Part model, mm, in its own coordinate system. Give positions to 0.01 mm unless a question says otherwise; leave off trailing zeros. Order: outer loops, then holes, each group sorted by start corner. A loop starts at its lowest first (then second) coordinate and runs counter-clockwise, first axis right, second up.
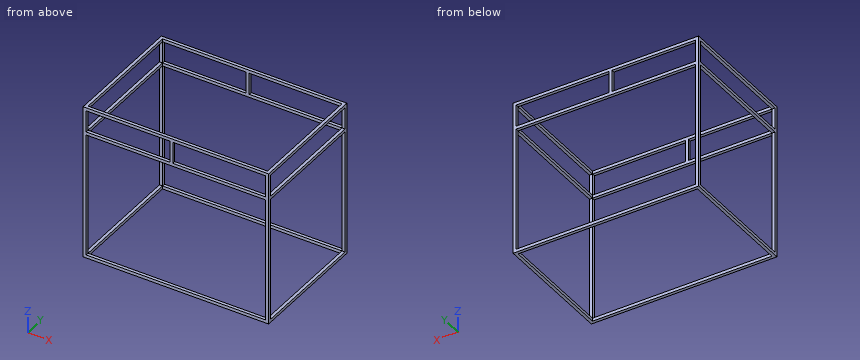
from build123d import *

# Parameters (mm, degrees)
SKETCH1_W               = 914.4
SKETCH1_H               = 609.6
SKETCH1_W_2             = 884.4
SKETCH1_H_2             = 579.6
BOSS_EXTRUDE2_DEPTH     = 762
SKETCH4_W               = 884.4
SKETCH4_H               = 609.6
SKETCH4_W_2             = 412.2
SKETCH4_H_2             = 107.4
SKETCH4_W_3             = 457.2
CUT_EXTRUDE3_DEPTH      = 762
CUT_EXTRUDE4_DEPTH      = 1374.291942344
CUT_EXTRUDE4_DEPTH_BACK = 1374.291942344
SKETCH5_W               = 107.4
SKETCH5_H               = 579.6
SKETCH5_W_2             = 609.6


with BuildPart() as part:
    # Sketch1 → Boss-Extrude2 (new body)
    with BuildSketch(Plane.XY):
        with Locations((479.545925455, 380.152114317)):
            Rectangle(SKETCH1_W, SKETCH1_H)
        with Locations((479.545925455, 380.152114317)):
            Rectangle(SKETCH1_W_2, SKETCH1_H_2, mode=Mode.SUBTRACT)
    extrude(amount=BOSS_EXTRUDE2_DEPTH)

    # Sketch4 → Cut-Extrude3 (cut)
    with BuildSketch(Plane(origin=(0, 75.352114317, 0), x_dir=(-1, 0, 0), z_dir=(0, -1, 0))):
        with Locations((-479.545925455, -319.8)):
            Rectangle(SKETCH4_W, SKETCH4_H)
        with Locations((-243.445925455, -693.3)):
            Rectangle(SKETCH4_W_2, SKETCH4_H_2)
        with Locations((-693.145925455, -693.3)):
            Rectangle(SKETCH4_W_3, SKETCH4_H_2)
    extrude(amount=-CUT_EXTRUDE3_DEPTH, mode=Mode.SUBTRACT)

    # Sketch5 → Cut-Extrude4 (cut, two sides: drawn at the far end of the back side and taken through both)
    with BuildSketch(Plane(origin=(936.745925455, 0, 0), x_dir=(0, 0, -1), z_dir=(1, 0, 0)).offset(-CUT_EXTRUDE4_DEPTH_BACK)):
        with Locations((-693.3, 380.152114317)):
            Rectangle(SKETCH5_W, SKETCH5_H)
        with Locations((-319.8, 380.152114317)):
            Rectangle(SKETCH5_W_2, SKETCH5_H)
    extrude(amount=CUT_EXTRUDE4_DEPTH + CUT_EXTRUDE4_DEPTH_BACK, mode=Mode.SUBTRACT)


solid = part.part
Item 1: Drop a flat-ended pin along its axis: P1, Ø16.5, axis at x = 926.5, y = 327.5, coming from the -Z side. Give the stop position or say it passes through.
Item 2: Band-saw the part on B-B on y = 244. List the corners of the cut face in (x, z), plus the area to 3 significant figures.
Item 3: Band-saw the part on C-C on z = 154. List the corners of the cut face in (x, y).
Item 4: Band-saw the part on A-A on x = 240.5. List the corners of the cut face in (y, z), plus the area to 3 significant figures.
Working result:
1. P1: stops at z = 0
2. outline: (22.35, 0) - (37.35, 0) - (37.35, 15) - (22.35, 15) - close; (22.35, 624.6) - (37.35, 624.6) - (37.35, 639.6) - (22.35, 639.6) - close; (22.35, 747) - (37.35, 747) - (37.35, 762) - (22.35, 762) - close; (921.75, 0) - (936.75, 0) - (936.75, 15) - (921.75, 15) - close; (921.75, 624.6) - (936.75, 624.6) - (936.75, 639.6) - (921.75, 639.6) - close; (921.75, 747) - (936.75, 747) - (936.75, 762) - (921.75, 762) - close
2. area: 1,350 mm2
3. outline: (22.35, 75.35) - (37.35, 75.35) - (37.35, 90.35) - (22.35, 90.35) - close; (22.35, 669.95) - (37.35, 669.95) - (37.35, 684.95) - (22.35, 684.95) - close; (921.75, 75.35) - (936.75, 75.35) - (936.75, 90.35) - (921.75, 90.35) - close; (921.75, 669.95) - (936.75, 669.95) - (936.75, 684.95) - (921.75, 684.95) - close
4. outline: (75.35, 0) - (90.35, 0) - (90.35, 15) - (75.35, 15) - close; (75.35, 624.6) - (90.35, 624.6) - (90.35, 639.6) - (75.35, 639.6) - close; (75.35, 747) - (90.35, 747) - (90.35, 762) - (75.35, 762) - close; (669.95, 0) - (684.95, 0) - (684.95, 15) - (669.95, 15) - close; (669.95, 624.6) - (684.95, 624.6) - (684.95, 639.6) - (669.95, 639.6) - close; (669.95, 747) - (684.95, 747) - (684.95, 762) - (669.95, 762) - close
4. area: 1,350 mm2
